Verification items for the finished model (mm, model axes). A direction names the side the tool comes from. Coordinates: 2 decimals unless noted, no trailing zeros. Order: outer loops, then holes, each group sorted by start corner. A loop starts at its lowest first (then second) coordinate and runs counter-clockwise, first axis right, second up.
Q1. Thickness scan on line 1 (X direction, y = 7, z = -13.5); line 2 (Y direction, x = 1, z = 3.5). Record the ranges inside material, lowest first.
Q2. Draft check along Y on faces 6 (the flat face through (-1, -25, 0)), 7 (the flat face through (33, -15, 0)), 8 (the flat face through (40, -20, 0)). Enter one of: pulls with the +Y half, pulls with the -Y half, needs draft (parallel to the pull), parting line crosses it, or undercut.
Q3. Cross-section at A-A, the plane x = -27.5. Record the boundary of the cut face in (y, z), and give its area (3 significant figures).
Q4. Set-up check for faces 1 (the flat face through (40, 20, 0)), 2 (the flat face through (0, 10, 0)), 3 (the flat face through (-1, 11, 15)), 4 (the flat face through (25, 0, 0)), 5 (the flat face through (-25, 0, 0)): record each of +Z, -Z, +X, -X, +Y, -Y from which the full face is reachable in a straight line by a thin tool's end or side.
Q5. Cross-section at B-B, the plane z = 10. Record the boundary of the cut face in (x, y), and give its area (3 significant figures).
Q6. Cross-section at D-D, the plane y = -13.5. Record the boundary of the cut face in (x, z).
Q7. Depth check by flat-ended pin: P1, Ø6, axis at y = 3.5, z = 2, coming from the +X side; P2, Ø10, axis at x = -3.5, y = -2.5, coming from the +Z side; P3, Ø9, axis at y = -0.5, z = 5, coming from the -X side. Enter the tip coordinate at first touch or a pass-through.
from build123d import *

# Parameters (mm, degrees)
SKETCH1_W           = 30
SKETCH1_H           = 20
BOSS_EXTRUDE1_DEPTH = 15


with BuildPart() as part:
    # Sketch1 → Boss-Extrude1 (new, symmetric)
    with BuildSketch(Plane.XY):
        Polygon((-40, 15), (-25, 15), (-25, -15), (-40, -15), (-40, -25), (40, -25), (40, -15), (25, -15), (25, 15), (40, 15), (40, 25), (-40, 25), align=None)
        Rectangle(SKETCH1_W, SKETCH1_H, mode=Mode.SUBTRACT)
    extrude(amount=BOSS_EXTRUDE1_DEPTH, both=True)


solid = part.part
Check values:
1. line 1: x = -25 to -15, 15 to 25
1. line 2: y = -25 to -10, 10 to 25
2. face 6: pulls with the -Y half
2. face 7: undercut
2. face 8: needs draft
3. outline: (-25, -15) - (-15, -15) - (-15, 15) - (-25, 15) - close; (15, -15) - (25, -15) - (25, 15) - (15, 15) - close
3. area: 600 mm2
4. face 1: +Z, -Z, +X, +Y, -Y
4. face 2: +Z, -Z
4. face 3: +Z, +X, -X, +Y, -Y
4. face 4: +Z, -Z, +X
4. face 5: +Z, -Z, -X
5. outline: (-40, -25) - (40, -25) - (40, -15) - (25, -15) - (25, 15) - (40, 15) - (40, 25) - (-40, 25) - (-40, 15) - (-25, 15) - (-25, -15) - (-40, -15) - close; hole (-15, -10) - (15, -10) - (15, 10) - (-15, 10) - close
5. area: 2,500 mm2
6. outline: (-25, -15) - (25, -15) - (25, 15) - (-25, 15) - close
7. P1: stops at x = 25
7. P2: passes through
7. P3: stops at x = -25
